Geometry: final body of the model. Coordinates: model frame, mm. A direction names the side the tool comes from. Round coordinates to 2 decimals unless told otherwise and drop trailing zeros. Loops run counter-clockwise (first coordinate to the right, second up) from the corner with the lowest first, then second, coordinate; pieces in that order, holes last. Notation, with made-up numbers: (-36, -34) - (-9, -34) arc R12 cw to (-9, -23) - close; hole circle Ø1 at (26, -16). An arc over 180 degrees is marked (long way). Answer as CSV lines item,"result".
from build123d import *

# Parameters (mm, degrees)
SKETCH_1_R      = 1.6
SKETCH_1_W      = 15
SKETCH_1_H      = 6
SKETCH_1_H_2    = 5
EXTRUDE_1_DEPTH = 3
FILLET_1_R      = 2
FILLET_2_R      = 3


with BuildPart() as part:
    # 草图1 → 凸台-拉伸1 (new body)
    with BuildSketch(Plane.XY):
        Polygon((0, 0), (0, 26.8), (14, 26.8), (14, 29.8), (24, 29.8), (24, 26.8), (34, 26.8), (34, 0), align=None)
        with Locations((3, 17)):
            Circle(SKETCH_1_R, mode=Mode.SUBTRACT)
        with Locations((3, 10)):
            Circle(SKETCH_1_R, mode=Mode.SUBTRACT)
        with Locations((29.2, 13.5)):
            Circle(SKETCH_1_R, mode=Mode.SUBTRACT)
        with Locations((22.5, 7)):
            Rectangle(SKETCH_1_W, SKETCH_1_H, mode=Mode.SUBTRACT)
        with Locations((22.5, 18.5)):
            Rectangle(SKETCH_1_W, SKETCH_1_H_2, mode=Mode.SUBTRACT)
    extrude(amount=EXTRUDE_1_DEPTH)

    # 圆角1
    fillet_1_edges = [part.edges().sort_by_distance(p)[0] for p in [
        (15, 10, 1.5),
        (15, 4, 1.5),
        (30, 4, 1.5),
        (30, 10, 1.5),
        (15, 21, 1.5),
        (15, 16, 1.5),
        (30, 16, 1.5),
        (30, 21, 1.5),
    ]]
    fillet(fillet_1_edges, radius=FILLET_1_R)

    # 圆角2
    fillet_2_edges = [part.edges().sort_by_distance(p)[0] for p in [
        (0, 0, 1.5),
        (34, 0, 1.5),
    ]]
    fillet(fillet_2_edges, radius=FILLET_2_R)


solid = part.part
(1) Section B-B (y = 13.5). Output: boundary loops of the cut face in (x, z).
Findings below:
outline,"(0, 0) - (27.6, 0) - (27.6, 3) - (0, 3) - close; (30.8, 0) - (34, 0) - (34, 3) - (30.8, 3) - close"
(2) Access query for faces 4 (the face through (29.4, 4.57, 1.52)), 5 (the face through (14, 28, 1)), 6 (the face through (29, 26.8, 1)). Directions: +Z, -Z, +X, -X, +Y, -Y. A direction counts if a zero-diameter tool reaches every point of the face in a straight line with its end or side. Return the directions, or none.
Findings below:
face 4,"+Z, -Z"
face 5,"+Z, -Z, -X, +Y"
face 6,"+Z, -Z, +X, +Y"
(3) Section A-A (x = 29.2). Output: boundary loops of the cut face in (y, z).
Findings below:
outline,"(0, 0) - (4.4, 0) - (4.4, 3) - (0, 3) - close; (9.6, 0) - (11.9, 0) - (11.9, 3) - (9.6, 3) - close; (15.1, 0) - (16.4, 0) - (16.4, 3) - (15.1, 3) - close; (20.6, 0) - (26.8, 0) - (26.8, 3) - (20.6, 3) - close"
(4) Material intervals for line 1 along Y through (x, z) = (23, 0.45); line 2 along Y through (x, z) = (3, 1.45); line 3 along X through (y, z) = (6.25, 2.2), sorted ascending.
Findings below:
line 1,"0 to 4, 10 to 16, 21 to 29.8"
line 2,"0 to 8.4, 11.6 to 15.4, 18.6 to 26.8"
line 3,"0 to 15, 30 to 34"
(5) Section D-D (z = 0.8). Give the number of separate pieces and of enclosed holes in the cut face, and give its area (3 significant figures).
Findings below:
separate pieces,"1"
enclosed holes,"5"
area,"755 mm2"
(6) Section C-C (x = 18). Output: boundary loops of the cut face in (y, z), and give its area (3 significant figures).
Findings below:
outline,"(0, 0) - (4, 0) - (4, 3) - (0, 3) - close; (10, 0) - (16, 0) - (16, 3) - (10, 3) - close; (21, 0) - (29.8, 0) - (29.8, 3) - (21, 3) - close"
area,"56.4 mm2"
(7) Pin query (flat end, axial travel): P1, Ø0.9, axis at x = 5, z = 1.5, coming from the +Y side; P2, Ø3, axis at x = 3, y = 17, coming from the -Z side; P3, Ø1.5, axis at y = 28.5, z = 1.5, coming from the +X side. Return the tip coordinate at first contact, or that it passes through.
Findings below:
P1,"y = 26.8"
P2,"through"
P3,"x = 24"
(8) Draft query along Y for faces 1 (the face through (34, 15, 1)), 2 (the face through (22, 16, 1)), 3 (the face through (0.86, 0.9, 1.52)). Return one class per face: pulls with the +Y half, pulls with the -Y half, needs draft (parallel to the pull), parting line crosses it, or undercut.
Findings below:
face 1,"needs draft"
face 2,"undercut"
face 3,"pulls with the -Y half"
